Read the model definition and answer for the solid it produces. Units are mm, in the model's axes. Face numbers are marked on the shaded views. Round coordinates to 2 decimals unless told otherwise and drop trailing zeros. Order: outer loops, then holes, each group sorted by start corner. A loop starts at its lowest first (then second) coordinate and runs counter-clockwise, first axis right, second up. Notation, with made-up numbers: (-21.75, 79) - (17.25, 79) arc R23 ccw to (17.25, 87) - close; hole circle Ø11 at (87, 25). An arc over 180 degrees is marked (long way). Put each result on its own line as item: value. Start each with the question number.
Q1. Each of these flat-tipped pins is pushed along its axis until it touches: pin 1 Ø1 at (x, y) = (25.5, -7) entering from -Z; pin 2 Ø10 at (x, z) = (-13.5, -9.5) entering from -Y; pin 3 Ø10.5 at (x, y) = (-11.5, -12.5) entering from -Z. Where does it stop, or does it pass through?
Q2. For a pull along Y with two mould halves and no side action, classify the marked faces 1, 2 and 3 as pulls with the +Y half, pulls with the -Y half, needs draft (parallel to the pull), parting line crosses it, or undercut.
Q3. Section D-D on y = -1.5 is taken. Give the vertices of the cut face in (x, z) (3 decimals).
Q4. Section C-C on z = -21 is taken. Give the vertices of the cut face in (x, y) (3 decimals), then the cut area to 3 significant figures.
Q5. Section B-B on y = -17.5 is taken. Give the vertices of the cut face in (x, z) (3 decimals), then the cut area to 3 significant figures.
Q6. Find the intervals of material crossed by line 1 along Y through (x, z) = (38.5, -12.75) (3 decimals); line 2 along X through (y, z) = (-2.75, -10.25) (3 decimals), in increasing order. Write a range as from..to.
from build123d import *

# Parameters (mm, degrees)
HIERRO_ANGULAR_1_X_1_X_0_125_1_DEPTH = 126.87
CROQUIS3_W                           = 3.25
CROQUIS3_H                           = 22.225
CORTAR_EXTRUIR1_DEPTH                = 10
CROQUIS4_W                           = 126.87
CROQUIS4_H                           = 4.4
CORTAR_EXTRUIR2_DEPTH                = 10
CHAFL_N1_SIZE                        = 2
CHAFL_N2_SIZE                        = 2


with BuildPart() as part:
    # Sketch1 → Hierro angular 1 X 1 X 0.125(1) (new body)
    with BuildSketch(Plane(origin=(-63.435, 0, 0), x_dir=(0, -1, 0), z_dir=(1, 0, 0))):
        with BuildLine():
            Line((0, 0), (0, 25.4))
            Line((0, 25.4), (0.00508, 25.4))
            ThreePointArc((0.00508, 25.4), (2.246551928, 24.471551928), (3.175, 22.23008))
            Line((3.175, 22.23008), (3.175, 7.9375))
            ThreePointArc((3.175, 7.9375), (4.569903955, 4.569903955), (7.9375, 3.175))
            Line((7.9375, 3.175), (22.23008, 3.175))
            ThreePointArc((22.23008, 3.175), (24.471551928, 2.246551928), (25.4, 0.00508))
            Line((25.4, 0.00508), (25.4, 0))
            Line((25.4, 0), (0, 0))
        make_face()
    extrude(amount=HIERRO_ANGULAR_1_X_1_X_0_125_1_DEPTH)

    # Croquis3 → Cortar-Extruir1 (cut)
    with BuildSketch(Plane(origin=(0, 0, 0), x_dir=(1, 0, 0), z_dir=(0, 1, 0))):
        with Locations((-61.81, 14.2875)):
            Rectangle(CROQUIS3_W, CROQUIS3_H)
        with Locations((61.81, 14.2875)):
            Rectangle(CROQUIS3_W, CROQUIS3_H)
    extrude(amount=-CORTAR_EXTRUIR1_DEPTH, mode=Mode.SUBTRACT)

    # Croquis4 → Cortar-Extruir2 (cut)
    with BuildSketch(Plane.XY):
        with Locations((0, -23.2)):
            Rectangle(CROQUIS4_W, CROQUIS4_H)
    extrude(amount=-CORTAR_EXTRUIR2_DEPTH, mode=Mode.SUBTRACT)

    # Chaflán1
    chafl_n1_edges = [part.edges().sort_by_distance(p)[0] for p in [
        (0, -21, 0),
    ]]
    chamfer(chafl_n1_edges, length=CHAFL_N1_SIZE)

    # Chaflán2
    chafl_n2_edges = [part.edges().sort_by_distance(p)[0] for p in [
        (63.435, -9.5, 0),
        (-63.435, -9.5, 0),
    ]]
    chamfer(chafl_n2_edges, length=CHAFL_N2_SIZE)


solid = part.part
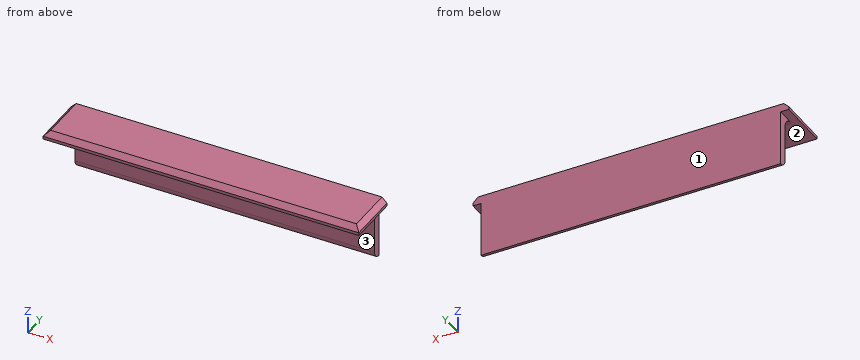
Findings:
1. pin 1: z = -3.4
1. pin 2: y = -4.64
1. pin 3: z = -3.22
2. face 1: pulls with the +Y half
2. face 2: needs draft
2. face 3: pulls with the -Y half
3. outline: (-63.435, -3.175) - (-60.185, -3.175) - (-60.185, -25.025) - (60.185, -25.025) - (60.185, -3.175) - (63.435, -3.175) - (63.435, -2) - (61.435, 0) - (-61.435, 0) - (-63.435, -2) - close
4. outline: (-60.185, -3.175) - (60.185, -3.175) - (60.185, 0) - (-60.185, 0) - close
4. area: 382 mm2
5. outline: (-63.435, -3.175) - (63.435, -3.175) - (63.435, -2) - (61.435, 0) - (-61.435, 0) - (-63.435, -2) - close
5. area: 399 mm2
6. line 1: -3.175..0
6. line 2: -60.185..60.185
